Read the model definition and answer for the solid it produces. Units are mm, in the model's axes. Face numbers are marked on the shaded views. Coordinates: 2 decimals unless noted, no trailing zeros. Order: outer loops, then holes, each group sorted by start corner. A loop starts at its lowest first (then second) coordinate and runs counter-clockwise, first axis right, second up. Notation, with made-up numbers: M -23.75,50.25 L -2.75,50.25 A16 cw -2.75,79.25 Z; hole C -9,26 d3. An arc over 180 degrees is marked long. Use a Markdown table: item, result. Add a question column.
1) Each of these flat-tipped pins is pushed along its axis until it touches: pin 1 Ø3 at (y, z) = (10.97, -19.07) entering from -X; pin 2 Ø6 at (x, z) = (4, 20) entering from -Y; pin 3 Ø1.2 at (x, z) = (7, 14) entering from -Y; pin 4 Ø8 at (x, z) = (8, -5) entering from -Y. Where does it stop, or does it pass through?
2) The mould has two halves that part along Z. Classify the marked faces 1, 2 and 3: released by +Z, released by -Z, zero draft, split by the parting line, or undercut.
3) Find section D-D on y = 22. Write down the section's boundary in (x, z).
4) Find section C-C on x = 13. Write down the section's boundary in (y, z), plus the area to 3 significant figures.
5) Find section B-B on z = -10.5. Write down the section's boundary in (x, y), plus the area to 3 significant figures.
6) Find section A-A on y = 0. Write down the section's boundary in (x, z), plus the area to 3 significant figures.
7) Find the intervals of material crossed by probe 1 along Y at (x, z) = (7, 0); probe 2 along Y at (x, z) = (20.5, 17.5); probe 3 along Z at (x, y) = (3, 11), in increasing order. Write a range as [from, to].
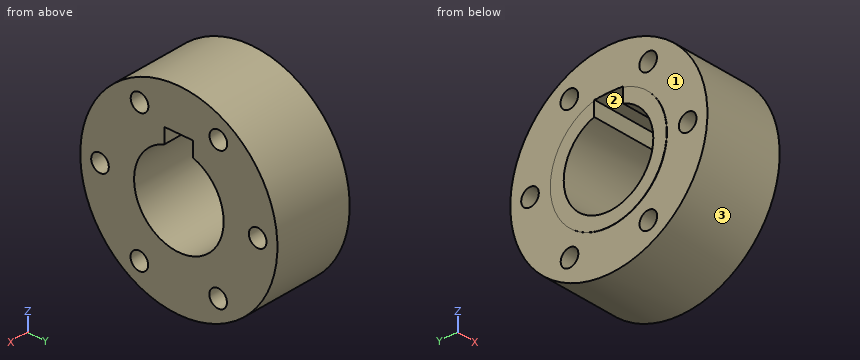
Autodesk Inventor part; units mm, degrees
ref_plane "YZ Plane" through (0, 0, 0) normal (1, 0, 0) x (0, 1, 0)
ref_plane "XZ Plane" through (0, 0, 0) normal (0, 1, 0) x (-1, 0, 0)
ref_plane "XY Plane" through (0, 0, 0) normal (0, 0, 1) x (1, 0, 0)
sketch "Skizze1" plane through (0, 0, 0) normal (1, 0, 0) x (0, 1, 0)
  circle A0 centre (0, 0) radius 12.5
  circle A1 centre (0, 0) radius 16.25
  dimension "d0" = 25
  dimension "d1" = 32.5
extrude "Extrusion1" add sketch "Skizze1" along normal mid plane 0.1
sketch "Skizze2" plane through (0.05, 0, 0) normal (1, 0, 0) x (0, 0, -1)
  circle A0 centre (0, 0) radius 27.5
  dimension "d5" = 55
extrude "Extrusion2" add sketch "Skizze2" along normal blind 22
sketch "Skizze4" plane through (22.05, 0, 0) normal (1, 0, 0) x (0, 0, -1)
  circle A0 centre (0, 0) radius 12.5
  dimension "d8" = 25
extrude "Extrusion3" cut sketch "Skizze4" against normal blind 30
sketch "Skizze5" plane through (0.05, 0, 0) normal (-1, 0, 0) x (0, 0, 1)
  point P0 (0, 0)
  point P1 (0.0333, -22)
  point P2 (19.0692, -10.9712)
  point P3 (19.0359, 11.0288)
  point P4 (-0.0333, 22)
  point P5 (-19.0692, 10.9712)
  point P6 (-19.0359, -11.0288)
  dimension "d18" = 22
  dimension "d21" = 360
hole "Bohrung1" at (0.05, -22, 0.0333) at (0.05, -10.9712, 19.0692) at (0.05, 11.0288, 19.0359) at (0.05, 22, -0.0333) at (0.05, 10.9712, -19.0692) at (0.05, -11.0288, -19.0359) direction (1, 0, 0) diameter 4.917 end through all
sketch "Skizze6" plane through (22.05, 0, 0) normal (1, 0, 0) x (0, 0, -1)
  line L0 (-16, -4) -> (-9, -4)
  line L1 (-9, -4) -> (-9, 4)
  line L2 (-9, 4) -> (-16, 4)
  line L3 (-16, 4) -> (-16, -4)
  circle A0 centre (0, 0) radius 12.5
  line L4 (-16, -4) -> (-9, 4) construction
  line L5 (-9, -4) -> (-16, 4) construction
  point P0 (-12.5, 0)
  point P1 (-11.8427, -4)
  point P2 (-11.8427, 4)
  dimension "d23" = 7
  dimension "d24" = 8
  dimension "d25" = 9
extrude "Extrusion4" cut sketch "Skizze6" against normal blind 52 contours L3 L2 A0 L0
properties part number "Befestigung bremsscheibe"
Check result:
| question | item | result |
|---|---|---|
| 1 | pin 1 | passes through |
| 1 | pin 2 | stops at y = -21.62 |
| 1 | pin 3 | stops at y = -24.01 |
| 1 | pin 4 | stops at y = -27.48 |
| 2 | face 1 | zero draft |
| 2 | face 2 | undercut |
| 2 | face 3 | split by the parting line |
| 3 | outline | M 0.05,-16.5 L 22.05,-16.5 L 22.05,-2.49 L 0.05,-2.49 Z; M 0.05,2.43 L 22.05,2.43 L 22.05,16.5 L 0.05,16.5 Z |
| 4 | outline | C 0,0 d55; hole C -22,0.03 d4.92; hole C -11.03,-19.04 d4.92; hole C -10.97,19.07 d4.92; hole M -4,11.84 A12.5 ccw long 4,11.84 L 4,16 L -4,16 Z; hole C 10.97,-19.07 d4.92; hole C 11.03,19.04 d4.92; hole C 22,-0.03 d4.92 |
| 4 | area | 1,740 mm2 |
| 5 | outline | M -0.05,-12.4 L 0.05,-12.4 L 0.05,-25.42 L 22.05,-25.42 L 22.05,-6.78 L -0.05,-6.78 Z; M -0.05,6.78 L 22.05,6.78 L 22.05,25.42 L 0.05,25.42 L 0.05,12.4 L -0.05,12.4 Z |
| 5 | area | 821 mm2 |
| 6 | outline | M -0.05,-16.25 L 0.05,-16.25 L 0.05,-27.5 L 22.05,-27.5 L 22.05,-12.5 L -0.05,-12.5 Z; M -0.05,16 L 22.05,16 L 22.05,27.5 L 0.05,27.5 L 0.05,16.25 L -0.05,16.25 Z |
| 6 | area | 583 mm2 |
| 7 | probe 1 | y = [-27.5, -24.46], [-19.54, -12.5], [12.5, 19.54], [24.46, 27.5] |
| 7 | probe 2 | y = [-21.21, -12.86], [-9.08, 9.11], [12.95, 21.21] |
| 7 | probe 3 | z = [-25.2, -21.53], [-16.61, -5.94], [5.94, 16.58], [21.49, 25.2] |
